Can you work these out from the model? Positions are in its coordinate system, mm. A direction names the side the tool comes from. Coordinates: 2 decimals unless noted, no trailing zeros. Loops run counter-clockwise (first coordinate to the right, second up) from the corner with the lowest first, then second, coordinate; pieces in that order, holes last. Notation, with made-up numbers: (89, -14.5) -> (109, -14.5) arc R8 ccw to (109, -8.5) -> close; hole circle Ø5 at (63, -13). An arc over 180 degrees is marked (long way). Use one line per item in the form item = value. Start each with the question number.
(1) Imagine slicing it at A-A (z = 0). List the corners of the cut face in (x, y) for me.
(2) I'm going to push flat-ended pins straight in: pin 1 (2 mm diameter, centred on x = -46.5, y = 1.5, fed in from -Z); pin 2 (4 mm diameter, centred on y = 1, z = 5, fed in from +X); pin 3 (1 mm diameter, centred on x = -54.5, z = -6.5, fed in from +Y). Where does each tip first touch, or does it pass through?
(3) Imagine slicing it at B-B (y = -0.25). List the corners of the cut face in (x, z) for me.
(4) I need wall thicknesses on line 1 (Y direction, x = -52.25, z = -6.5); line 2 (Z direction, x = -53, y = 3.75); line 3 (X direction, y = 1.75, z = -1.5). Which ranges of each line are inside material? Lowest first, please. Write a range as [from, to].
(5) Thinking about a two-plate mould opening in X: for faces 3 (the flat face through (-41, 4, 0)), 4 (the cylindrical face through (-56.224, 1.972, -1.734)), 5 (the flat face through (-46, 1, 1.1)), which applies, released by +X, released by -X, zero draft, split by the parting line, or undercut?
(6) Imagine slicing it at C-C (y = 1.5). List the corners of the cut face in (x, z) for me.
(7) On a 3-axis mill with a long thin cutter (end or side, diameter ignored), from which of +Z, -Z, +X, -X, +Y, -Y can I reach the whole of each face in a straight line? I mean faces 1 (the cylindrical face through (-45.737, -1.972, 0.351)), 2 (the conical face through (-49.62, 1.17, 5.44)). Say none if no direction works.
```python
from build123d import *

# Parameters (mm, degrees)
SKETCH1_R           = 8
BOSS_EXTRUDE3_DEPTH = 4
SKETCH5_R           = 6.6
CUT_EXTRUDE2_DEPTH  = 3
CUT_EXTRUDE2_DRAFT  = -20
SKETCH6_R           = 2.7
BOSS_EXTRUDE4_DEPTH = 4
SKETCH7_R           = 2.15
CUT_EXTRUDE3_DEPTH  = 6
CUT_EXTRUDE3_DRAFT  = -2
FILLET1_R           = 0.5


with BuildPart() as part:
    # Sketch1 → Boss-Extrude3 (new body)
    with BuildSketch(Plane(origin=(0, 0, 0), x_dir=(1, 0, 0), z_dir=(0, 1, 0))):
        with Locations(Location((-48.414322475, 0, 0), (0, 0, 270))):
            Circle(SKETCH1_R)
    extrude(amount=BOSS_EXTRUDE3_DEPTH)


with BuildPart() as cut_extrude2_tool:
    # Sketch5 → Cut-Extrude2 (with draft: the straight prism first)
    with BuildSketch(Plane(origin=(0, 4, 0), x_dir=(1, 0, 0), z_dir=(0, 1, 0))):
        with Locations((-48.414322475, 0)):
            Circle(SKETCH5_R)
    extrude(amount=-CUT_EXTRUDE2_DEPTH)
    # Cut-Extrude2: the draft: its side faces are tilted about the plane it starts from
    cut_extrude2_sides = [cut_extrude2_tool.faces().sort_by_distance(p)[0] for p in [
        (-55.014322475, 2.5, 0),
    ]]
    draft(cut_extrude2_sides, Plane(origin=(0, 4, 0), x_dir=(1, 0, 0), z_dir=(0, 1, 0)), CUT_EXTRUDE2_DRAFT)


with BuildPart() as part_1:
    add(part.part)

    # Cut-Extrude2: cut by cut_extrude2_tool
    add(cut_extrude2_tool.part, mode=Mode.SUBTRACT)

    # Sketch6 → Boss-Extrude4 (add)
    with BuildSketch(Plane.XZ):
        with Locations(Location((-48.414322475, 0, 0), (0, 0, 270))):
            Circle(SKETCH6_R)
    extrude(amount=BOSS_EXTRUDE4_DEPTH)


with BuildPart() as cut_extrude3_tool:
    # Sketch7 → Cut-Extrude3 (with draft: the straight prism first)
    with BuildSketch(Plane.XZ.offset(4)):
        with Locations((-48.414322475, 0)):
            Circle(SKETCH7_R)
    extrude(amount=-CUT_EXTRUDE3_DEPTH)
    # Cut-Extrude3: the draft: its side faces are tilted about the plane it starts from
    cut_extrude3_sides = [cut_extrude3_tool.faces().sort_by_distance(p)[0] for p in [
        (-50.564322475, -1, 0),
    ]]
    draft(cut_extrude3_sides, Plane.XZ.offset(4), CUT_EXTRUDE3_DRAFT)


with BuildPart() as part_2:
    add(part_1.part)

    # Cut-Extrude3: cut by cut_extrude3_tool
    add(cut_extrude3_tool.part, mode=Mode.SUBTRACT)

    # Fillet1
    fillet1_edges = [part_2.edges().sort_by_distance(p)[0] for p in [
        (-50.389718627, 1, 0),
        (-50.564322475, -4, 0),
        (-55.014322475, 4, 0),
    ]]
    fillet(fillet1_edges, radius=FILLET1_R)


solid = part_2.part
```
Worked out:
q1.outline = (-56.41, 0) -> (-51.11, 0) -> (-51.11, -4) -> (-51.05, -4) arc R0.5 ccw to (-50.55, -3.52) -> (-50.41, 0.48) arc R0.5 ccw to (-50.91, 1) -> (-53.92, 1) -> (-54.89, 3.67) arc R0.5 ccw to (-55.36, 4) -> (-56.41, 4) -> close; (-46.42, 0.48) -> (-46.28, -3.52) arc R0.5 ccw to (-45.78, -4) -> (-45.71, -4) -> (-45.71, 0) -> (-40.41, 0) -> (-40.41, 4) -> (-41.46, 4) arc R0.5 ccw to (-41.93, 3.67) -> (-42.91, 1) -> (-45.92, 1) arc R0.5 ccw to start
q2.pin_1 = -7.95
q2.pin_2 = -41
q2.pin_3 = through
q3.outline = circle Ø5.4 at (-48.41, 0); hole circle Ø4.04 at (-48.41, 0)
q4.line_1 = [0, 4]
q4.line_2 = [-6.56, -4.63], [4.63, 6.56]
q4.line_3 = [-56.27, -54], [-42.83, -40.56]
q5.face_3 = zero draft
q5.face_4 = split by the parting line
q5.face_5 = undercut
q6.outline = circle Ø16 at (-48.41, 0); hole circle Ø11.38 at (-48.41, 0)
q7.face_1 = -Y
q7.face_2 = +Y
